from build123d import *

# Parameters (mm, degrees)
F1_T     = -2
F2_R     = 28
F3_DEPTH = 25


with BuildPart() as f4:
    # F0 (on Front) → F4 (revolve)
    with BuildSketch(Plane.XZ):
        Polygon((47.7527889609, 0), (47.7527889609, 30), (-12.2472110391, 30), (-22.2472110391, 25), (-77.1310710907, 25), (-77.1310710907, 0), align=None)
    revolve(axis=Axis((-5.2267275751, 0, 0), (1, 0, 0)))

    # F1
    f1_openings = [f4.faces().sort_by_distance(p)[0] for p in [
        (-77.131071, 0, 0),
    ]]
    offset(amount=F1_T, openings=f1_openings, kind=Kind.INTERSECTION)

    # F2 (on face) → F3 (cut)
    with BuildSketch(Plane(origin=(45.7527889609, 0, 0), x_dir=(0, -1, 0), z_dir=(-1, 0, 0))):
        Circle(F2_R)
    extrude(amount=-F3_DEPTH, mode=Mode.SUBTRACT)


solid = f4.part
Build history of the part. All positions in model axes, mm. Give positions to 0.01 mm unless a question says otherwise; leave off trailing zeros. Order: outer loops, then holes, each group sorted by start corner. A loop starts at its lowest first (then second) coordinate and runs counter-clockwise, first axis right, second up. Notation, with made-up numbers: M 72.25,76.25 L 127.25,76.25 A7 ccw 127.25,82.25 Z; hole C 12,45.25 d10. An arc over 180 degrees is marked long. Use one line per item in the form item = value.
Q1. Slice it at C-C, the plane x = -40. Write the cut outline in (y, z).
Conclusion:
outline = C 0,0 d50; hole C 0,0 d46
Q2. Slice it at A-A, the plane z = 0. Write the cut outline in (x, y).
Conclusion:
outline = M -77.13,-25 L -22.25,-25 L -12.25,-30 L 47.75,-30 L 47.75,-28 L -11.78,-28 L -21.78,-23 L -77.13,-23 Z; M -77.13,23 L -21.78,23 L -11.78,28 L 47.75,28 L 47.75,30 L -12.25,30 L -22.25,25 L -77.13,25 Z
Q3. Slice it at D-D, the plane x = 35. Write the cut outline in (y, z), and give its area (3 significant figures).
Conclusion:
outline = C 0,0 d60; hole C 0,0 d56
area = 364 mm2
Q4. Pull direction Z, two halves, no side cores. Call faces 1 (the flat face through (-77.131, 7.3, 22.1)), 2 (the conical face through (-21.29, -6.98, 22.17)), 3 (the cylindrical face through (-50.073, -7.509, 23.846)): released by +Z, released by -Z, zero draft, split by the parting line, or undercut.
Conclusion:
face_1 = zero draft
face_2 = undercut
face_3 = split by the parting line
Q5. Wall check: probe 1 along Z at (x, y) = (11, 0); probe 2 along Y at (x, z) = (-53.5, 0); probe 3 along Z at (x, y) = (-61.5, -1). Give the ranges that are in metal, low to high.
Conclusion:
probe_1 = -30 to -28, 28 to 30
probe_2 = -25 to -23, 23 to 25
probe_3 = -24.98 to -22.98, 22.98 to 24.98
Q6. Pin check, flat tips, straight feed: P1, Ø5, axis at x = -3.5, z = -10, coming from the -Y side; P2, Ø12, axis at x = -44.5, y = 11.5, coming from the -Z side; P3, Ø5, axis at x = -46.5, y = 14, coming from the -Z side. Stop position of each tip, or through.
Conclusion:
P1 = -29.05
P2 = -24.39
P3 = -22.2
